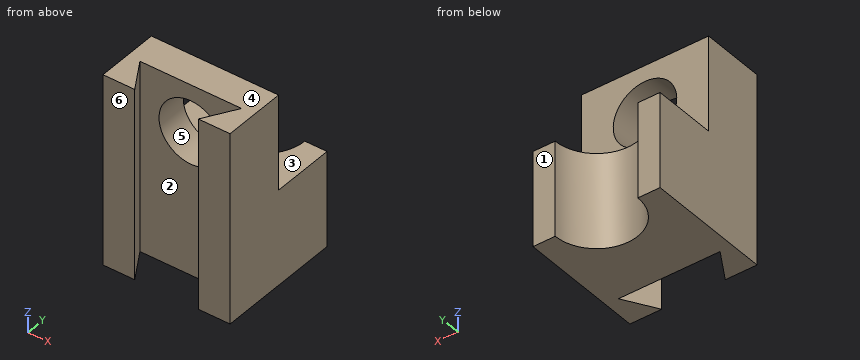
from build123d import *

# Parameters (mm, degrees)
EXTRUDE_1_DEPTH     = 20
CUT_EXTRUDE_2_DEPTH = 75.833147735
SKETCH_3_R          = 10
CUT_EXTRUDE_3_DEPTH = 67.332495807
CUT_EXTRUDE_4_DEPTH = 54.851648071


with BuildPart() as part:
    # 草图1 → 凸台-拉伸1 (new, symmetric)
    with BuildSketch(Plane(origin=(0, 0, 0), x_dir=(0, 0, -1), z_dir=(1, 0, 0))):
        Polygon((0, 0), (0, 20), (30, 20), (30, 40), (60, 40), (60, 0), align=None)
    extrude(amount=EXTRUDE_1_DEPTH, both=True)

    # 草图2 → 切除-拉伸2 (cut, through all)
    with BuildSketch(Plane.XY):
        Polygon((10, 0), (16, 10), (-16, 10), (-10, 0), align=None)
    extrude(amount=-CUT_EXTRUDE_2_DEPTH, mode=Mode.SUBTRACT)

    # 草图3 → 切除-拉伸3 (cut, through all)
    with BuildSketch(Plane(origin=(0, 20, 0), x_dir=(1, 0, 0), z_dir=(0, 1, 0))):
        with Locations(Location((0, 15, 0), (0, 0, 270))):
            Circle(SKETCH_3_R)
    extrude(amount=-CUT_EXTRUDE_3_DEPTH, mode=Mode.SUBTRACT)

    # 草图4 → 切除-拉伸4 (cut, through all)
    with BuildSketch(Plane.XY.offset(-30)):
        with BuildLine():
            Line((-13, 40), (13, 40))
            ThreePointArc((13, 40), (0, 27), (-13, 40))
        make_face()
    extrude(amount=-CUT_EXTRUDE_4_DEPTH, mode=Mode.SUBTRACT)


solid = part.part
Work out the finished part from the listing and answer in its coordinate system (mm). Face numbers are marked on the shaded views. A direction names the side the tool comes from. Coordinates: 2 decimals unless noted, no trailing zeros. Write each loop counter-clockwise with the first axis right and the second up, starting at its lowest first coordinate (ties: lowest second). Pieces come first, ordered by that corner, then holes. Notation, with made-up numbers: M 13,-3.75 L 68,-3.75 A31 cw 68,24.25 Z; hole C 35.5,65.5 d3. An arc over 180 degrees is marked long. Use one line per item in the form item = value. Start each with the question number.
1. A tool of negligible diameter and unlimited length cuts with its end or side. For the marked faces 1, 2 and 3, from which of +Z, -Z, +X, -X, +Y, -Y can it reach the whole face along a straight path? Write none if from no direction.
2. The part is cut by section B-B (z = -15). Give the vertices of the cut face in (x, y).
3. Each of these flat-tipped pins is pushed along its axis until it touches: P1, Ø9, axis at x = 0, z = -13.5, coming from the +Y side; P2, Ø16, axis at x = 4, z = -23.5, coming from the -Y side; P3, Ø10, axis at x = 8.5, y = 30, coming from the +Z side; P4, Ø8, axis at x = -0.5, z = -52, coming from the +Y side. Where does it stop, or does it pass through?
4. The mould has two halves that part along Z. Classify the marked faces 4, 5 and 6: released by +Z, released by -Z, zero draft, split by the parting line, or undercut.
5. The part is cut by section A-A (x = 0). Give the vertices of the cut face in (y, z), plus the area to 3 significant figures.
6. Straight lines are drawn through the part: probe 1 along X at (y, z) = (12.75, -15); probe 2 along Z at (x, y) = (-11, 23.5); probe 3 along Z at (x, y) = (-2, 14.5). For each, find the intervals that lie inside material, in ascending order. Write a range as from..to.
7. The part is cut by section C-C (y = 7). Give the vertices of the cut face in (x, z).
8. The part is cut by section D-D (y = 12.5). Give the vertices of the cut face in (x, z).
Evaluation:
q1.face_1 = +Z, -Z, +X, -X, +Y
q1.face_2 = +Z, -Z
q1.face_3 = +Z, +X, -X, +Y
q2.outline = M -20,0 L -10,0 L -16,10 L -10,10 L -10,20 L -20,20 Z; M 10,0 L 20,0 L 20,20 L 10,20 L 10,10 L 16,10 Z
q3.P1 = through
q3.P2 = 0
q3.P3 = -30
q3.P4 = 27.8
q4.face_4 = released by +Z
q4.face_5 = undercut
q4.face_6 = zero draft
q5.outline = M 10,-60 L 27,-60 L 27,-30 L 20,-30 L 20,-25 L 10,-25 Z; M 10,-5 L 20,-5 L 20,0 L 10,0 Z
q5.area = 610 mm^2
q6.probe_1 = -20..-10, 10..20
q6.probe_2 = -60..-30
q6.probe_3 = -60..-24.8, -5.2..0
q7.outline = M -20,-60 L -14.2,-60 L -14.2,0 L -20,0 Z; M 14.2,-60 L 20,-60 L 20,0 L 14.2,0 Z
q8.outline = M -20,-60 L 20,-60 L 20,0 L -20,0 Z; hole C 0,-15 d20
